```python
from build123d import *

# Parameters (mm, degrees)
SKETCH1_W                                    = 15
SKETCH1_H                                    = 55
BOSS_EXTRUDE1_DEPTH                          = 4
CSK_FOR_M4_HEX_SOCKET_COUNTERSUNK_HE_2_COUNT = 2
CSK_FOR_M4_HEX_SOCKET_COUNTERSUNK_HE_2_PITCH = 20
SKETCH15_W                                   = 12
SKETCH15_H                                   = 18
BOSS_EXTRUDE2_DEPTH                          = 5


with BuildPart() as part:
    # Sketch1 → Boss-Extrude1 (new body)
    with BuildSketch(Plane.XY):
        Rectangle(SKETCH1_W, SKETCH1_H)
    extrude(amount=BOSS_EXTRUDE1_DEPTH)

    # Sketch5 → CSK for M4 Hex Socket Countersunk Head Screw1 (revolve, cut)
    with BuildSketch(Plane(origin=(-0.5, 0.5, 0), x_dir=(0, 1, 0), z_dir=(1, 0, 0))):
        Polygon((0, 0), (0, 4), (2.275, 4), (2.25, 3.975), (2.25, 2.34), (4.59, 0), align=None)
    csk_for_m4_hex_socket_countersunk_head_s = revolve(axis=Axis((-0.5, 0.5, -6.35), (0, 0, 1)), mode=Mode.SUBTRACT)

    # CSK for M4 Hex Socket Countersunk He 2: CSK for M4 Hex Socket Countersunk Head Screw1 ×2
    with Locations(*[(0, -i * CSK_FOR_M4_HEX_SOCKET_COUNTERSUNK_HE_2_PITCH, 0) for i in range(1, CSK_FOR_M4_HEX_SOCKET_COUNTERSUNK_HE_2_COUNT)]):
        add(csk_for_m4_hex_socket_countersunk_head_s, mode=Mode.SUBTRACT)

    # Sketch15 → Boss-Extrude2 (add)
    with BuildSketch(Plane(origin=(0, 0, 0), x_dir=(-1, 0, 0), z_dir=(0, 0, -1))):
        with Locations((0.7, 18.5)):
            Rectangle(SKETCH15_W, SKETCH15_H)
    extrude(amount=BOSS_EXTRUDE2_DEPTH)

    # Sketch19 → M3 Clearance Hole1 (revolve, cut)
    with BuildSketch(Plane(origin=(-3.7, 24.85, -5), x_dir=(0, 1, 0), z_dir=(1, 0, 0))):
        Polygon((0, 0), (0, 9), (1.625, 9), (1.6, 8.975), (1.6, 0), align=None)
    revolve(axis=Axis((-3.7, 24.85, -11.35), (0, 0, 1)), mode=Mode.SUBTRACT)


solid = part.part
```
Input: part model. Units: mm. Frame: model coordinates. A direction names the side the tool comes from. Round coordinates to 2 decimals unless told otherwise and drop trailing zeros. Order: outer loops, then holes, each group sorted by start corner. A loop starts at its lowest first (then second) coordinate and runs counter-clockwise, first axis right, second up. Notation, with made-up numbers: (26, -10.5) - (52, -10.5) arc R20 cw to (52, 28.5) - close; hole circle Ø1 at (-11, 82). An arc over 180 degrees is marked (long way). Answer in a Markdown table with one row per item.
Item 1: Line query: line 1 (Y direction, x = -0.5, z = 3.15); line 2 (X direction, y = 24.85, z = -2.5); line 3 (X direction, y = 0.5, z = 3.65). Output: solid intervals per line, ascending.
Model answer:
| item | result |
|---|---|
| line 1 | y = -27.5 to -21.75, -17.25 to -1.75, 2.75 to 27.5 |
| line 2 | x = -6.7 to -5.3, -2.1 to 5.3 |
| line 3 | x = -7.5 to -2.75, 1.75 to 7.5 |
Item 2: Reachability of faces 1 (the flat face through (-1, 9.5, -2)), 2 (the flat face through (0, 27.5, -1)), 3 (the flat face through (-6.7, 18, -2)), 4 (the flat face through (5.3, 18, -2)), 5 (the conical face through (-1.22, -17.21, 2.19)) from +Z, -Z, +X, -X, +Y, -Y: full face, straight path, thin tool, end or side. Return the list, or none.
Model answer:
| item | result |
|---|---|
| face 1 | -Z, +X, -X, -Y |
| face 2 | +Z, -Z, +X, -X, +Y |
| face 3 | -Z, -X, +Y, -Y |
| face 4 | -Z, +X, +Y, -Y |
| face 5 | -Z |
Item 3: Section query A-A (y = 0.5). Return the cut outline in (x, z) (3 decimals), then the cut area to 3 significant figures.
Model answer:
| item | result |
|---|---|
| outline | (-7.5, 0) - (-5.09, 0) - (-2.75, 2.34) - (-2.75, 3.975) - (-2.775, 4) - (-7.5, 4) - close; (1.75, 2.34) - (4.09, 0) - (7.5, 0) - (7.5, 4) - (1.775, 4) - (1.75, 3.975) - close |
| area | 36.5 mm² |
Item 4: Pin query (flat end, axial travel): pin 1 (6 mm diameter, centred on x = -0.5, y = 0.5, fed in from +Z); pin 2 (6 mm diameter, centred on x = -0.5, y = -19.5, fed in from -Z); pin 3 (3 mm diameter, centred on x = 3.5, y = -21.5, fed in from -Z); pin 4 (1.5 mm diameter, centred on y = 15.5, z = -2.5, fed in from -X). Return the tip coordinate at first contact, or that it passes through.
Model answer:
| item | result |
|---|---|
| pin 1 | stops at z = 4 |
| pin 2 | stops at z = 1.59 |
| pin 3 | stops at z = 0 |
| pin 4 | stops at x = -6.7 |
Item 5: Section query C-C (z = 3). Return the cut outline in (x, y).
Model answer:
| item | result |
|---|---|
| outline | (-7.5, -27.5) - (7.5, -27.5) - (7.5, 27.5) - (-7.5, 27.5) - close; hole circle Ø3.2 at (-3.7, 24.85); hole circle Ø4.5 at (-0.5, -19.5); hole circle Ø4.5 at (-0.5, 0.5) |
Item 6: Mould query, pull axis Y, two halves, no side actions, for faces 6 (the cylindrical face through (0.869, -1.286, 3.146)), 7 (the flat face through (7.5, 0, 2)), 8 (the flat face through (0, -27.5, 2)). Classes: released by +Y, released by -Y, zero draft, split by the parting line, or undercut.
Model answer:
| item | result |
|---|---|
| face 6 | undercut |
| face 7 | zero draft |
| face 8 | released by -Y |
Item 7: Section query D-D (y = 18.5). Return the cut outline in (x, z).
Model answer:
| item | result |
|---|---|
| outline | (-7.5, 0) - (-6.7, 0) - (-6.7, -5) - (5.3, -5) - (5.3, 0) - (7.5, 0) - (7.5, 4) - (-7.5, 4) - close |
Item 8: Section query B-B (z = -3). Return the cut outline in (x, y), then the cut area to 3 significant figures.
Model answer:
| item | result |
|---|---|
| outline | (-6.7, 9.5) - (5.3, 9.5) - (5.3, 27.5) - (-6.7, 27.5) - close; hole circle Ø3.2 at (-3.7, 24.85) |
| area | 208 mm² |
